Geometry check sheet. Reference: the model listing, model coordinates, mm. A direction names the side the tool comes from. Give positions to 0.01 mm unless a question says otherwise; leave off trailing zeros. Loops run counter-clockwise (first coordinate to the right, second up) from the corner with the lowest first, then second, coordinate; pieces in that order, holes last.
1. Tool access check on faces 5 (the flat face through (-35, 0, -20)), 6 (the flat face through (-20, 11.035, -20)), 7 (the flat face through (-11, 20, -20)). Record the directions out of +Z, -Z, +X, -X, +Y, -Y that give a thin tool (end or side, any length) a straight path to the whole face; none if there is none.
2. Go/stop test with flat-tipped pins: pin 1 Ø1 at (x, y) = (-24.5, 34.5) entering from +Z; pin 2 Ø6 at (x, z) = (-18.5, -29.5) entering from -Y; pin 3 Ø5 at (y, z) = (30.5, -16.5) entering from +X. Record where each tip stops, or that it passes through.
3. Material ranges on L1, parallel to X at y = 7, z = -23.5; L2, parallel to Y at x = -13, z = -10; L3, parallel to Y at x = -24, z = -23, recorded low to high.
4. Cross-section at C-C, the plane z = -20. Record the cut outline in (x, y), plus the area to 3 significant figures.
5. Cross-section at D-D, the plane y = 35. Record the cut outline in (x, z).
6. Cross-section at B-B, the plane x = -20. Record the cut outline in (y, z), plus the area to 3 significant figures.
7. Release check for a two-part mould opening along X. For faces 1 (the flat face through (-30, 5, -20)), 2 (the flat face through (-40, 10, -20)), 3 (the flat face through (-10, 5, -20)), 4 (the flat face through (-5, 0, -20)) record: +X half, -X half, draft (parallel to the pull), parting line (faces both ways), or undercut.
8. Cross-section at A-A, the plane y = 10. Record the cut outline in (x, z).
from build123d import *

# Parameters (mm, degrees)
SKETCH1_W           = 40
SKETCH1_H           = 40
BOSS_EXTRUDE1_DEPTH = 20
SKETCH2_W           = 20
SKETCH2_H           = 11.035436779
CUT_EXTRUDE1_DEPTH  = 61
SKETCH3_R           = 7.76528749
BOSS_EXTRUDE2_DEPTH = 20


with BuildPart() as part:
    # Sketch1 → Boss-Extrude1 (new body)
    with BuildSketch(Plane(origin=(0, 0, 0), x_dir=(1, 0, 0), z_dir=(0, 1, 0))):
        with Locations((-20, 20)):
            Rectangle(SKETCH1_W, SKETCH1_H)
    extrude(amount=BOSS_EXTRUDE1_DEPTH)

    # Sketch2 → Cut-Extrude1 (cut, through all)
    with BuildSketch(Plane.XY):
        with Locations((-20, 5.51771839)):
            Rectangle(SKETCH2_W, SKETCH2_H)
    extrude(amount=-CUT_EXTRUDE1_DEPTH, mode=Mode.SUBTRACT)

    # Sketch3 → Boss-Extrude2 (add)
    with BuildSketch(Plane(origin=(0, 20, 0), x_dir=(1, 0, 0), z_dir=(0, 1, 0))):
        with Locations(Location((-20, 20, 0), (0, 0, 270))):
            Circle(SKETCH3_R)
    extrude(amount=BOSS_EXTRUDE2_DEPTH)


solid = part.part
Result:
1. face 5: +Z, -Z, +X, -X, -Y
1. face 6: +Z, -Z, -Y
1. face 7: +Y
2. pin 1: stops at z = -13.34
2. pin 2: stops at y = 11.04
2. pin 3: stops at x = -12.3
3. L1: x = -40 to -30, -10 to 0
3. L2: y = 11.04 to 20
3. L3: y = 11.04 to 40
4. outline: (-40, 0) - (-30, 0) - (-30, 11.04) - (-10, 11.04) - (-10, 0) - (0, 0) - (0, 20) - (-12.23, 20) - (-12.23, 40) - (-27.77, 40) - (-27.77, 20) - (-40, 20) - close
4. area: 890 mm2
5. outline: circle Ø15.53 at (-20, -20)
6. outline: (11.04, -40) - (20, -40) - (20, -27.77) - (40, -27.77) - (40, -12.23) - (20, -12.23) - (20, 0) - (11.04, 0) - close
6. area: 669 mm2
7. face 1: undercut
7. face 2: -X half
7. face 3: undercut
7. face 4: draft
8. outline: (-40, -40) - (-30, -40) - (-30, 0) - (-40, 0) - close; (-10, -40) - (0, -40) - (0, 0) - (-10, 0) - close
